from build123d import *

# Parameters (mm, degrees)
SKETCH_1_R          = 64
SKETCH_1_R_2        = 63.5
EXTRUDE_1_DEPTH     = 25
CUT_EXTRUDE_1_DEPTH = 2000


with BuildPart() as part:
    # 草图1 → 凸台-拉伸1 (new body)
    with BuildSketch(Plane.XY):
        Circle(SKETCH_1_R)
        Circle(SKETCH_1_R_2, mode=Mode.SUBTRACT)
    extrude(amount=EXTRUDE_1_DEPTH)

    # 草图2 → 切除-拉伸1 (cut)
    with BuildSketch(Plane(origin=(0, 0, 0), x_dir=(0, 0, -1), z_dir=(1, 0, 0))):
        with BuildLine():
            Line((-14.5, -0.75), (-12.5, -0.75))
            Line((-12.5, -0.75), (-12.5, 0.75))
            Line((-12.5, 0.75), (-14.5, 0.75))
            ThreePointArc((-14.5, 0.75), (-15.25, 0), (-14.5, -0.75))
        make_face()
    extrude(amount=-CUT_EXTRUDE_1_DEPTH, mode=Mode.SUBTRACT)


solid = part.part
Can you work these out from the model? Positions are in its coordinate system, mm. Give positions to 0.01 mm unless a question says otherwise; leave off trailing zeros. Loops run counter-clockwise (first coordinate to the right, second up) from the corner with the lowest first, then second, coordinate; pieces in that order, holes last. Notation, with made-up numbers: (80.5, 70) -> (131.5, 70) arc R26 cw to (131.5, 108) -> close; hole circle Ø10 at (66, 80.5). An arc over 180 degrees is marked (long way). Use one line per item in the form item = value.
1) We'd pull the mould along X, two halves only. Please class faces 1 (the face through (-13.77, -61.99, 12.32)), 2 (the face through (-13.87, -62.48, 12.32)): released by +X, released by -X, zero draft, split by the parting line, or undercut.
Answers:
face_1 = undercut
face_2 = split by the parting line
2) Will these pins go through, and if not, where does the flat tip stop? pin 1 (3 mm diameter, centred on x = -32, z = 10.5, fed in from +Y) (3 decimals); pin 2 (8 mm diameter, centred on y = 7, z = 15, fed in from +X); pin 3 (8 mm diameter, centred on x = 9.5, z = 16, fed in from -Y); pin 4 (8 mm diameter, centred on y = -2, z = 13, fed in from +X).
Answers:
pin_1 = 56.265
pin_2 = 63.93
pin_3 = -63.76
pin_4 = 64
3) If we section it at C-C (z = 4): Please give me the cut outline in (x, y).
Answers:
outline = circle Ø128 at (0, 0); hole circle Ø127 at (0, 0)
4) I need wall thicknesses on line 1 along X through (y, z) = (0, 17); line 2 along X through (y, z) = (53, 11.5) (3 decimals). Which ranges of each line are inside material? Lowest first, please.
Answers:
line_1 = -64 to -63.5, 63.5 to 64
line_2 = -35.875 to -34.975, 34.975 to 35.875
5) If we section it at A-A (x = 0): Please give me the cut outline in (y, z).
Answers:
outline = (-64, 0) -> (-63.5, 0) -> (-63.5, 25) -> (-64, 25) -> close; (63.5, 0) -> (64, 0) -> (64, 25) -> (63.5, 25) -> close
6) If we section it at B-B (y = 26.5): Please give me the cut outline in (x, z).
Answers:
outline = (-58.26, 0) -> (-57.71, 0) -> (-57.71, 25) -> (-58.26, 25) -> close; (57.71, 0) -> (58.26, 0) -> (58.26, 25) -> (57.71, 25) -> close
